```python
from build123d import *

# Parameters (mm, degrees)
DODANIE_WYCI_GNI_CIE1_DEPTH                       = 8
WYTNIJ_WYCI_GNI_CIE1_DEPTH                        = 8
WYTNIJ_WYCI_GNI_CIE2_DEPTH                        = 39.052595181
WYTNIJ_WYCI_GNI_CIE2_DEPTH_BACK                   = 39.052595181
OTWORY_USTALAJ_CE_5_0MM1_D                        = 5
OTWORY_USTALAJ_CE_5_0MM1_DEPTH                    = 20
OTWORY_USTALAJ_CE_5_0MM1_TIP                      = 1.502151548
SZKIC8_R                                          = 3.15
WYTNIJ_WYCI_GNI_CIE3_DEPTH                        = 10
ZAOKR_GLENIE1_R                                   = 1
POG_BIENIE_WALCOWE_POD_M5_RUB_Z_BEM_W_D           = 5.5
POG_BIENIE_WALCOWE_POD_M5_RUB_Z_BEM_W_DEPTH       = 44
POG_BIENIE_WALCOWE_POD_M5_RUB_Z_BEM_W_CBORE_D     = 10
POG_BIENIE_WALCOWE_POD_M5_RUB_Z_BEM_W_CBORE_DEPTH = 5
POG_BIENIE_WALCOWE_POD_M5_RUB_Z_BEM_W_TIP         = 1.652366702
SZKIC11_R                                         = 3.25
WYTNIJ_WYCI_GNI_CIE4_DEPTH                        = 44.174066359


with BuildPart() as part:
    # Szkic1 → Dodanie-wyciągnięcie1 (new, symmetric)
    with BuildSketch(Plane.XY):
        Polygon((0, 0), (8, 0), (8, 30), (13, 30), (22, 15), (22, -20), (0, -20), align=None)
    dodanie_wyci_gni_cie1 = extrude(amount=DODANIE_WYCI_GNI_CIE1_DEPTH, both=True)

    # Lustro1: Dodanie-wyciągnięcie1 across plane
    add(dodanie_wyci_gni_cie1.mirror(Plane(origin=(0, -20, 8), x_dir=(0, 0, 1), z_dir=(1, 0, 0))))

    # Szkic2 → Wytnij-wyciągnięcie1 (cut)
    with BuildSketch(Plane.XY.offset(8)):
        with BuildLine():
            Line((-13, -20), (13, -20))
            ThreePointArc((13, -20), (0, -7), (-13, -20))
        make_face()
    extrude(amount=-WYTNIJ_WYCI_GNI_CIE1_DEPTH, mode=Mode.SUBTRACT)

    # Szkic3 → Wytnij-wyciągnięcie2 (cut, two sides: drawn at the far end of the back side and taken through both)
    with BuildSketch(Plane.XY.offset(-WYTNIJ_WYCI_GNI_CIE2_DEPTH_BACK)):
        with BuildLine():
            ThreePointArc((9, -20), (0, -11), (-9, -20))
            Line((-9, -20), (9, -20))
        make_face()
    extrude(amount=WYTNIJ_WYCI_GNI_CIE2_DEPTH + WYTNIJ_WYCI_GNI_CIE2_DEPTH_BACK, mode=Mode.SUBTRACT)

    # Otwory ustalające Ø5.0mm1
    with Locations(Plane(origin=(0, -20, 0), x_dir=(-1, 0, 0), z_dir=(0, -1, 0))):
        with Locations((-17.5, 0), (17.5, 0)):
            Hole(OTWORY_USTALAJ_CE_5_0MM1_D / 2, depth=OTWORY_USTALAJ_CE_5_0MM1_DEPTH)
            with Locations((0, 0, -(OTWORY_USTALAJ_CE_5_0MM1_DEPTH + OTWORY_USTALAJ_CE_5_0MM1_TIP / 2))):  # 118° drill point
                Cone(0, OTWORY_USTALAJ_CE_5_0MM1_D / 2, OTWORY_USTALAJ_CE_5_0MM1_TIP, mode=Mode.SUBTRACT)

    # Szkic8 → Wytnij-wyciągnięcie3 (cut)
    with BuildSketch(Plane(origin=(0, -20, 0), x_dir=(-1, 0, 0), z_dir=(0, -1, 0))):
        with Locations(Location((17.5, 0, 0), (0, 0, 180))):
            Circle(SZKIC8_R)
        with Locations(Location((-17.5, 0, 0), (0, 0, 180))):
            Circle(SZKIC8_R)
    extrude(amount=-WYTNIJ_WYCI_GNI_CIE3_DEPTH, mode=Mode.SUBTRACT)

    # Zaokrąglenie1
    zaokr_glenie1_edges = [part.edges().sort_by_distance(p)[0] for p in [
        (8, 30, 0),
        (22, -2.5, 8),
        (13, 30, 0),
        (22, 15, 0),
        (17.5, 22.5, 8),
        (10.5, 30, 8),
        (-8, 15, 8),
        (-10.5, 30, 8),
        (-8, 30, 0),
        (-17.5, 22.5, 8),
        (-13, 30, 0),
        (-22, -2.5, 8),
        (-22, 15, 0),
        (-22, -2.5, -8),
        (8, 15, 8),
        (-17.5, 22.5, -8),
        (-10.5, 30, -8),
        (-8, 15, -8),
        (0, 0, 8),
        (0, -11, 0),
        (0, -11, -8),
        (0, 0, -8),
        (8, 15, -8),
        (10.5, 30, -8),
        (17.5, 22.5, -8),
        (22, -2.5, -8),
    ]]
    fillet(zaokr_glenie1_edges, radius=ZAOKR_GLENIE1_R)

    # Pogłębienie walcowe pod M5 Śrubę z łbem walcowym z gniazdem2
    with Locations(Plane(origin=(22, 156, 204.349537134), x_dir=(0, 0, -1), z_dir=(1, 0, 0))):
        with Locations((204.349537134, -149), (204.349537134, -137)):
            CounterBoreHole(POG_BIENIE_WALCOWE_POD_M5_RUB_Z_BEM_W_D / 2, POG_BIENIE_WALCOWE_POD_M5_RUB_Z_BEM_W_CBORE_D / 2, POG_BIENIE_WALCOWE_POD_M5_RUB_Z_BEM_W_CBORE_DEPTH, depth=POG_BIENIE_WALCOWE_POD_M5_RUB_Z_BEM_W_DEPTH)
            with Locations((0, 0, -(POG_BIENIE_WALCOWE_POD_M5_RUB_Z_BEM_W_DEPTH + POG_BIENIE_WALCOWE_POD_M5_RUB_Z_BEM_W_TIP / 2))):  # 118° drill point
                Cone(0, POG_BIENIE_WALCOWE_POD_M5_RUB_Z_BEM_W_D / 2, POG_BIENIE_WALCOWE_POD_M5_RUB_Z_BEM_W_TIP, mode=Mode.SUBTRACT)

    # Szkic11 → Wytnij-wyciągnięcie4 (cut, through all)
    with BuildSketch(Plane(origin=(-8, 0, 0), x_dir=(0, 0, -1), z_dir=(1, 0, 0))):
        with Locations((0, 7)):
            Circle(SZKIC11_R)
        with Locations((0, 19)):
            Circle(SZKIC11_R)
    extrude(amount=-WYTNIJ_WYCI_GNI_CIE4_DEPTH, mode=Mode.SUBTRACT)


solid = part.part
```
The listing builds one solid part. Answer for the finished solid, in the listing's coordinates (mm). A direction names the side the tool comes from. Coordinates: 2 decimals unless noted, no trailing zeros. Write each loop counter-clockwise with the first axis right and the second up, starting at its lowest first coordinate (ties: lowest second). Pieces come first, ordered by that corner, then holes. Notation, with made-up numbers: (21, 86.5) - (29, 86.5) arc R24 cw to (29, 98.5) - close; hole circle Ø9 at (-1, 89). An arc over 180 degrees is marked (long way). One line per item, written item: value.
1) Find section D-D (z = 6.25). Give the vertices of the cut face in (x, y).
Geometry check:
outline: (-22, -20) - (-13, -20) arc R13 cw to (13, -20) - (22, -20) - (22, 14.72) arc R1 ccw to (21.86, 15.24) - (13.29, 29.51) arc R1 ccw to (12.43, 30) - (9, 30) arc R1 ccw to (8, 29) - (8, 0) - (-8, 0) - (-8, 29) arc R1 ccw to (-9, 30) - (-12.43, 30) arc R1 ccw to (-13.29, 29.51) - (-21.86, 15.24) arc R1 ccw to (-22, 14.72) - close
2) Find section A-A (y = -8). Give the vertices of the cut face in (x, z).
Geometry check:
outline: (-22, -7) arc R1 ccw to (-21, -8) - (21, -8) arc R1 ccw to (22, -7) - (22, 7) arc R1 ccw to (21, 8) - (5, 8) - (5, 0) - (-5, 0) - (-5, 8) - (-21, 8) arc R1 ccw to (-22, 7) - close; hole circle Ø5 at (-17.5, 0); hole circle Ø5 at (17.5, 0)
3) Find section C-C (x = -11). Give the vertices of the cut face in (y, z).
Geometry check:
outline: (-20, -8) - (29, -8) arc R1 ccw to (30, -7) - (30, 7) arc R1 ccw to (29, 8) - (-13.07, 8) - (-13.07, 0) - (-20, 0) - close; hole circle Ø6.5 at (7, 0); hole circle Ø6.5 at (19, 0)
4) For a pull along Z with two mould halves and no side action, classify faces 1 (the flat face through (8, 14, 0)), 2 (the cylindrical face through (12.437, 4.315, -0.596)), 3 (the cylindrical face through (-17.38, 22.12, 7.71)) as pulls with the +Z half, pulls with the -Z half, needs draft (parallel to the pull), parting line crosses it, or undercut.
Geometry check:
face 1: needs draft
face 2: undercut
face 3: pulls with the +Z half
5) A tool of negligible diameter and unlimited length cuts with its end or side. For faces 4 (the cylindrical face through (15, -5, 0)), 5 (the cylindrical face through (-13.192, 15.827, 0.705)), 6 (the cylindrical face through (19.535, 11.957, 0.651)), 7 (the cylindrical face through (0, -7, 4)), from which of +Z, -Z, +X, -X, +Y, -Y can it reach the whole face along a straight path? Write none if from no direction.
Geometry check:
face 4: -Y
face 5: -X
face 6: +X
face 7: +Z, -Y
6) Find section B-B (y = 7). Give the vertices of the cut face in (x, z).
Geometry check:
outline: (-22, -7) arc R1 ccw to (-21, -8) - (-9, -8) arc R1 ccw to (-8, -7) - (-8, -3.25) - (-22, -3.25) - close; (-22, 3.25) - (-8, 3.25) - (-8, 7) arc R1 ccw to (-9, 8) - (-21, 8) arc R1 ccw to (-22, 7) - close; (8, -7) arc R1 ccw to (9, -8) - (21, -8) arc R1 ccw to (22, -7) - (22, -5) - (17, -5) - (17, -2.75) - (8, -2.75) - close; (8, 2.75) - (17, 2.75) - (17, 5) - (22, 5) - (22, 7) arc R1 ccw to (21, 8) - (9, 8) arc R1 ccw to (8, 7) - close
7) Each of these flat-tipped pins is pushed along its axis until it touches: pin 1 Ø7 at (x, z) = (17.5, 0) entering from +Y; pin 2 Ø4 at (x, z) = (-17.5, 0) entering from +Y; pin 3 Ø6.5 at (x, z) = (17.5, 0) entering from +Y. Where does it stop, or does it pass through?
Geometry check:
pin 1: stops at y = 28.33
pin 2: stops at y = 25.83
pin 3: stops at y = 27.92
8) Consider line 1 along X through (y, z) = (14, -3); line 2 along Z through (x, y) = (17.5, -6.5); line 3 along Z through (x, y) = (-16, 19). Determine where each line is inside the solid, lowest interval first. Write a range as from..to.
Geometry check:
line 1: x = -22..-8, 8..22
line 2: z = -8..-2.5, 2.5..8
line 3: z = -8..-3.25, 3.25..8
